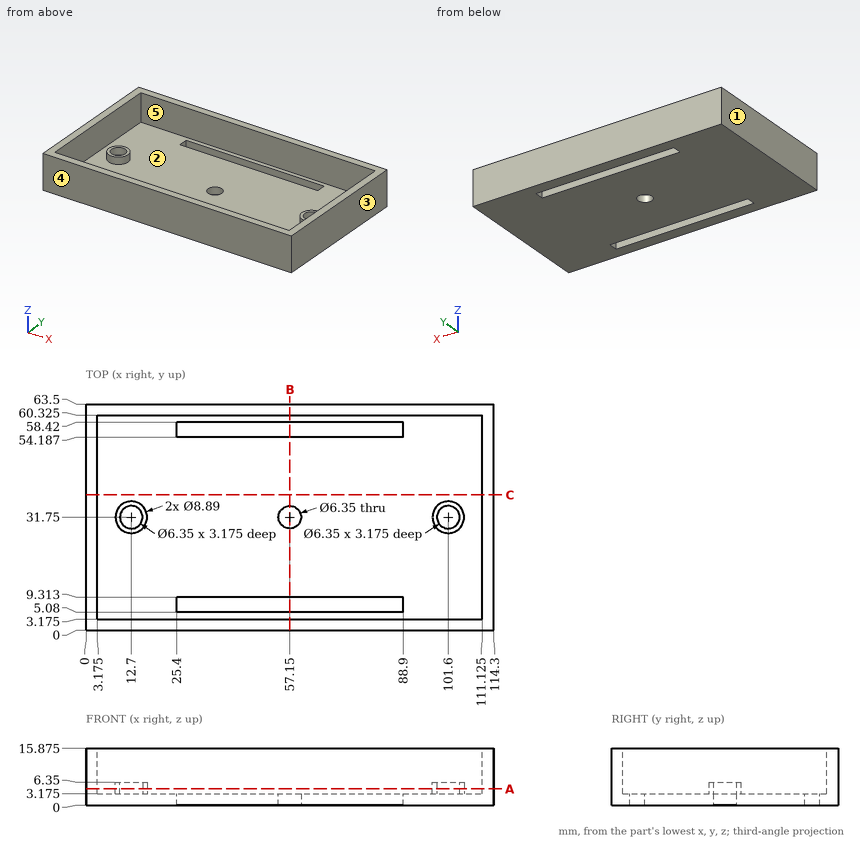
Drawing for the job (mm, zero at the part's lowest x, y, z). A direction names the side the tool comes from. Give positions to 0.01 mm unless a question says otherwise; leave off trailing zeros. Order: outer loops, then holes, each group sorted by start corner. A loop starts at its lowest first (then second) coordinate and runs counter-clockwise, first axis right, second up. Notation, with made-up numbers: M 48.5,10.25 L 76.5,10.25 A22 ccw 76.5,25.25 Z; hole C 39.5,4.25 d5. An arc over 180 degrees is marked long. Write item = value, one per line. Start each with the question number.
(1) Which spindle directions (+Z, -Z, +X, -X, +Y, -Y) get a long thin tool onto all of the face, cutting with end or side? Do the marked faces 4 and 5. Say none if no direction does.
(2) Probe L1, parallel to Y at x = 57.15, z = 1.55 (1 decimal); L2, parallel to Y at x = 12.7, z = 5.1 (1 decimal); L3, parallel to X at y = 49, z = 3.5 (1 decimal). List the from-to ranges inside material, lowest first. Write a range as [from, to].
(3) Slice it at A-A on z = 4.5. State how many separate pieces and enclosed holes the cut face has, plus the area to 3 significant figures.
(4) Slice it at C-C on y = 38. Write the cut outline in (x, z) (1 decimal).
(5) Pin check, flat tips, straight feed: pin 1 Ø3 at (x, y) = (100.5, 31) entering from +Z (3 decimals); pin 2 Ø4.5 at (x, y) = (99.5, 30.5) entering from +Z. Stop position of each tip, or through.
(6) Two-plate mould, pull along X, no slides. Class the marked faces 1, 2 and 3: released by +X, released by -X, zero draft, split by the parting line, or undercut.
(7) Slice it at B-B on x = 57.15. Write the cut outline in (y, z) (1 decimal), plus the area to 3 significant figures.
Responses:
q1.face_4 = +Z, -Z, +X, -X, -Y
q1.face_5 = +Z
q2.L1 = [0, 5.1], [9.3, 28.6], [34.9, 54.2], [58.4, 63.5]
q2.L2 = [0, 3.2], [27.3, 28.6], [34.9, 36.2], [60.3, 63.5]
q2.L3 = [0, 3.2], [111.1, 114.3]
q3.separate_pieces = 3
q3.enclosed_holes = 3
q3.area = 1,150 mm2
q4.outline = M 0,0 L 114.3,0 L 114.3,15.9 L 111.1,15.9 L 111.1,3.2 L 3.2,3.2 L 3.2,15.9 L 0,15.9 Z
q5.pin_1 = 3.175
q5.pin_2 = 6.35
q6.face_1 = released by -X
q6.face_2 = undercut
q6.face_3 = released by +X
q7.outline = M 0,0 L 5.1,0 L 5.1,3.2 L 3.2,3.2 L 3.2,15.9 L 0,15.9 Z; M 9.3,0 L 28.6,0 L 28.6,3.2 L 9.3,3.2 Z; M 34.9,0 L 54.2,0 L 54.2,3.2 L 34.9,3.2 Z; M 58.4,0 L 63.5,0 L 63.5,15.9 L 60.3,15.9 L 60.3,3.2 L 58.4,3.2 Z
q7.area = 235 mm2
